```python
from build123d import *

# Parameters (mm, degrees)
CROQUIS1_W              = 20
CROQUIS1_H              = 5.5
CROQUIS1_R              = 1
SALIENTE_EXTRUIR1_DEPTH = 0.45
CROQUIS2_W              = 11.5
CROQUIS2_H              = 5.5
SALIENTE_EXTRUIR2_DEPTH = 5
CROQUIS3_W              = 3
CROQUIS3_H              = 3
SALIENTE_EXTRUIR3_DEPTH = 1.5


with BuildPart() as part:
    # Croquis1 → Saliente-Extruir1 (new body)
    with BuildSketch(Plane(origin=(0, 0, 0), x_dir=(1, 0, 0), z_dir=(0, 1, 0))):
        Rectangle(CROQUIS1_W, CROQUIS1_H)
        with Locations(Location((-7.5, 0, 0), (0, 0, 270))):
            Circle(CROQUIS1_R, mode=Mode.SUBTRACT)
        with Locations(Location((7.5, 0, 0), (0, 0, 270))):
            Circle(CROQUIS1_R, mode=Mode.SUBTRACT)
    extrude(amount=SALIENTE_EXTRUIR1_DEPTH)

    # Croquis2 → Saliente-Extruir2 (add)
    with BuildSketch(Plane.XZ):
        Rectangle(CROQUIS2_W, CROQUIS2_H)
    extrude(amount=SALIENTE_EXTRUIR2_DEPTH)

    # Croquis3 → Saliente-Extruir3 (add)
    with BuildSketch(Plane(origin=(0, 0.45, 0), x_dir=(1, 0, 0), z_dir=(0, 1, 0))):
        with Locations((-2.774167271, 0)):
            Rectangle(CROQUIS3_W, CROQUIS3_H)
    extrude(amount=SALIENTE_EXTRUIR3_DEPTH)


solid = part.part
```
Part model, mm, in its own coordinate system. A direction names the side the tool comes from. Round coordinates to 2 decimals unless told otherwise and drop trailing zeros. Order: outer loops, then holes, each group sorted by start corner. A loop starts at its lowest first (then second) coordinate and runs counter-clockwise, first axis right, second up. Notation, with made-up numbers: M 64.5,32.25 L 97.5,32.25 A11 ccw 97.5,37.25 Z; hole C 57.25,25.25 d4. An arc over 180 degrees is marked long. Put each result on its own line as item: value. Start each with the question number.
1. Tool access for faces 1 (the face through (9, 0, 0)), 2 (the face through (-3, 1, -1.5)), 3 (the face through (-3, 1, 1.5)), 4 (the face through (-5.75, -2, 0)): list every direction of +Z, -Z, +X, -X, +Y, -Y with a clear straight run to the whole face (end or side of a thin tool).
2. Drill centre lines: probe 1 along X at (y, z) = (0.35, 0); probe 2 along Y at (x, z) = (-4.5, -1.9); probe 3 along X at (y, z) = (-1.25, 0.35). Where is each one in solid material? Low to high. Write a range as [from, to].
3. Two-plate mould, pull along X, no slides. Class faces 5 (the face through (-6.51, 0.22, -0.13)), 6 (the face through (-3, 1.95, 0)), 7 (the face through (8.49, 0.22, -0.13)), 8 (the face through (-4.274, 1, 0)): +X half, -X half, draft (parallel to the pull), parting line (faces both ways), or undercut.
4. Slice it at B-B on z = -0.8. List the corners of the cut face in (x, y), then the cut area to 3 significant figures.
5. Slice it at D-D on y = 0.25. List the corners of the cut face in (x, z), then the cut area to 3 significant figures.
6. Slice it at A-A on x = 7.5. List the corners of the cut face in (y, z).
7. Drop flat-ended pins along their axis: pin 1 (1.8 mm diameter, centred on x = -7.5, z = 0, fed in from +Y); pin 2 (2 mm diameter, centred on x = -8, z = -1, fed in from -Y); pin 3 (2.5 mm diameter, centred on y = -3.5, z = -1, fed in from -X); pin 4 (0.8 mm diameter, centred on x = -3, y = 1, fed in from +Z). Give the stop position or say it passes through.
8. Slice it at C-C on x = -4. List the corners of the cut face in (y, z), then the cut area to 3 significant figures.
Findings:
1. face 1: +Z, -Z, +X, -Y
1. face 2: -Z, +X, -X, +Y
1. face 3: +Z, +X, -X, +Y
1. face 4: +Z, -Z, -X, -Y
2. probe 1: [-10, -8.5], [-6.5, 6.5], [8.5, 10]
2. probe 2: [-5, 0.45]
2. probe 3: [-5.75, 5.75]
3. face 5: undercut
3. face 6: draft
3. face 7: undercut
3. face 8: -X half
4. outline: M -10,0 L -8.1,0 L -8.1,0.45 L -10,0.45 Z; M -6.9,0 L -5.75,0 L -5.75,-5 L 5.75,-5 L 5.75,0 L 6.9,0 L 6.9,0.45 L -1.27,0.45 L -1.27,1.95 L -4.27,1.95 L -4.27,0.45 L -6.9,0.45 Z; M 8.1,0 L 10,0 L 10,0.45 L 8.1,0.45 Z
4. area: 69.9 mm2
5. outline: M -10,-2.75 L 10,-2.75 L 10,2.75 L -10,2.75 Z; hole C -7.5,0 d2; hole C 7.5,0 d2
5. area: 104 mm2
6. outline: M 0,-2.75 L 0.45,-2.75 L 0.45,-1 L 0,-1 Z; M 0,1 L 0.45,1 L 0.45,2.75 L 0,2.75 Z
7. pin 1: through
7. pin 2: y = 0
7. pin 3: x = -5.75
7. pin 4: z = 1.5
8. outline: M -5,-2.75 L 0.45,-2.75 L 0.45,-1.5 L 1.95,-1.5 L 1.95,1.5 L 0.45,1.5 L 0.45,2.75 L -5,2.75 Z
8. area: 34.5 mm2
